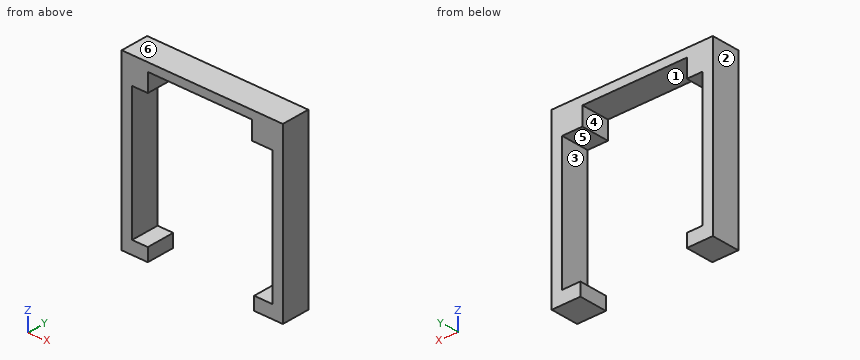
from build123d import *

# Parameters (mm, degrees)
BOX003_W     = 20
BOX003_H     = 26
BOX003_DEPTH = 3.5
BOX002_W     = 20.4
BOX002_H     = 25.4
BOX002_DEPTH = 10
BOX001_W     = 26.9
BOX001_H     = 26
BOX001_DEPTH = 25.4
BOX_W        = 30.9
BOX_H        = 5.4
BOX_DEPTH    = 33


with BuildPart() as cableslot:
    # Box003 → Box003 (new body)
    with BuildSketch(Plane(origin=(5, 0, 27.9), x_dir=(1, 0, 0), z_dir=(0, 0, 1))):
        with Locations((10, 13)):
            Rectangle(BOX003_W, BOX003_H)
    extrude(amount=BOX003_DEPTH)


with BuildPart() as gap:
    # Box002 → Box002 (new body)
    with BuildSketch(Plane(origin=(5, 0, 0), x_dir=(1, 0, 0), z_dir=(0, 0, 1))):
        with Locations((10.2, 12.7)):
            Rectangle(BOX002_W, BOX002_H)
    extrude(amount=BOX002_DEPTH)


with BuildPart() as bar:
    # Box001 → Box001 (new body)
    with BuildSketch(Plane(origin=(2, 0, 2.5), x_dir=(1, 0, 0), z_dir=(0, 0, 1))):
        with Locations((13.45, 13)):
            Rectangle(BOX001_W, BOX001_H)
    extrude(amount=BOX001_DEPTH)


with BuildPart() as cut002:
    # Box → Box (new body)
    with BuildSketch(Plane.XY):
        with Locations((15.45, 2.7)):
            Rectangle(BOX_W, BOX_H)
    extrude(amount=BOX_DEPTH)

    # Cut: cut Bar
    add(bar.part, mode=Mode.SUBTRACT)

    # Cut001: cut Gap
    add(gap.part, mode=Mode.SUBTRACT)

    # Cut002: cut CableSlot
    add(cableslot.part, mode=Mode.SUBTRACT)


with BuildPart() as cut002_1:
    # Cut002 placement: moved
    add(cut002.part.moved(Location((0, 0, 30))))


solid = cut002_1.part
Geometry check sheet. Reference: the model listing, model coordinates, mm. Face numbers are marked on the shaded views. A direction names the side the tool comes from. Give positions to 0.01 mm unless a question says otherwise; leave off trailing zeros. Loops run counter-clockwise (first coordinate to the right, second up) from the corner with the lowest first, then second, coordinate; pieces in that order, holes last.
(1) Depth check by flat-ended pin: pin 1 Ø1.5 at (x, y) = (20, 2.5) entering from -Z. Enter the tip coordinate at first touch or a pass-through.
From the geometry:
pin 1: stops at z = 61.4
(2) Thickness scan on L1, parallel to X at y = 4.45, z = 55; L2, parallel to X at y = 0.5, z = 32; L3, parallel to Z at x = 3, y = 0.4. Record the ranges inside material, lowest first.
From the geometry:
L1: x = 0 to 2, 28.9 to 30.9
L2: x = 0 to 5, 25.4 to 30.9
L3: z = 30 to 32.5, 57.9 to 63
(3) Release check for a two-part mould opening along Z. For the marked faces 1, 2 and 3 record: released by +Z, released by -Z, zero draft, split by the parting line, or undercut.
From the geometry:
face 1: released by -Z
face 2: zero draft
face 3: undercut
(4) Set-up check for the marked faces 4, 5 and 6: record each of +Z, -Z, +X, -X, +Y, -Y from which the full face is reachable in a straight line by a thin tool's end or side.
From the geometry:
face 4: -Z, +Y, -Y
face 5: +Y, -Y
face 6: +Z, +X, -X, +Y, -Y
(5) Section check D-D on x = 14.5. Record the cut outline in (y, z).
From the geometry:
outline: (0, 61.4) - (5.4, 61.4) - (5.4, 63) - (0, 63) - close
(6) Section check B-B on z = 35.5. Record the cut outline in (x, y).
From the geometry:
outline: (0, 0) - (2, 0) - (2, 5.4) - (0, 5.4) - close; (28.9, 0) - (30.9, 0) - (30.9, 5.4) - (28.9, 5.4) - close
(7) Section check A-A on x = 4.5. Record the cut outline in (y, z), then the cut area to 3 significant figures.
From the geometry:
outline: (0, 30) - (5.4, 30) - (5.4, 32.5) - (0, 32.5) - close; (0, 57.9) - (5.4, 57.9) - (5.4, 63) - (0, 63) - close
area: 41.0 mm2
(8) Section check C-C on y = 4.85. Record the cut outline in (x, z).
From the geometry:
outline: (0, 30) - (5, 30) - (5, 32.5) - (2, 32.5) - (2, 57.9) - (5, 57.9) - (5, 61.4) - (25, 61.4) - (25, 57.9) - (28.9, 57.9) - (28.9, 32.5) - (25.4, 32.5) - (25.4, 30) - (30.9, 30) - (30.9, 63) - (0, 63) - close
